from build123d import *
from build123d.topology import SkipClean

# Parameters (mm, degrees)
SKETCH2_W           = 56
SKETCH2_H           = 61
BOSS_EXTRUDE1_DEPTH = 2
SKETCH3_W           = 46
SKETCH3_H           = 53
BOSS_EXTRUDE4_DEPTH = 2
SKETCH4_W           = 61
SKETCH4_H           = 4
BOSS_EXTRUDE5_DEPTH = 1
SKETCH5_W           = 6
SKETCH5_H           = 7
SKETCH5_R           = 1.6
BOSS_EXTRUDE7_DEPTH = 4
CUT_EXTRUDE1_DEPTH  = 1
CHAMFER1_SIZE       = 7
CHAMFER2_SIZE       = 7
CHAMFER3_SIZE       = 7
SKETCH11_R          = 3.1
CUT_EXTRUDE3_DEPTH  = 2
CHAMFER5_SIZE       = 1
BOSS_EXTRUDE8_DEPTH = 4
SKETCH13_W          = 45.8
SKETCH13_H          = 52.8
CUT_EXTRUDE4_DEPTH  = 2
CHAMFER6_SIZE       = 0.5
SKETCH14_W          = 2.229283504
SKETCH14_H          = 1.6
CUT_EXTRUDE5_DEPTH  = 0.4
CHAMFER7_SIZE       = 0.4
SKETCH15_W          = 42.8
SKETCH15_H          = 20
CUT_EXTRUDE6_DEPTH  = 2
SKETCH17_W          = 105.377924995
SKETCH17_H          = 90.385080266
SKETCH17_W_2        = 45.7
SKETCH17_H_2        = 52.7
CUT_EXTRUDE7_DEPTH  = 2
FILLET1_R           = 3
FILLET2_R           = 1


with BuildPart() as part:
    # Sketch2 → Boss-Extrude1 (new, symmetric)
    with BuildSketch(Plane(origin=(0, 0, 0), x_dir=(1, 0, 0), z_dir=(0, 1, 0))):
        with Locations((-16.78535262, 5.61968945)):
            Rectangle(SKETCH2_W, SKETCH2_H)
    extrude(amount=BOSS_EXTRUDE1_DEPTH, both=True)

    # Sketch3 → Boss-Extrude4 (add)
    with BuildSketch(Plane(origin=(0, 2, 0), x_dir=(1, 0, 0), z_dir=(0, 1, 0))):
        with Locations((-15.78535262, 5.61968945)):
            Rectangle(SKETCH3_W, SKETCH3_H)
    extrude(amount=BOSS_EXTRUDE4_DEPTH)

    # Sketch4 → Boss-Extrude5 (add)
    with BuildSketch(Plane.ZY.offset(44.78535262)):
        with Locations((-5.61968945, 0)):
            Rectangle(SKETCH4_W, SKETCH4_H)
    extrude(amount=BOSS_EXTRUDE5_DEPTH)

    # Sketch5 → Boss-Extrude7 (add)
    # profile 1 of 4: a face of its own
    with BuildSketch(Plane.XZ.offset(2)):
        with Locations((0.21464738, -39.61968945)):
            Rectangle(SKETCH5_W, SKETCH5_H)
        with Locations(Location((0.21464738, -39.61968945, 0), (0, 0, 270))):
            Circle(SKETCH5_R, mode=Mode.SUBTRACT)
    # profile 2 of 4: a face of its own
    with BuildSketch(Plane.XZ.offset(2)):
        with Locations((-34.78535262, -39.61968945)):
            Rectangle(SKETCH5_W, SKETCH5_H)
        with Locations(Location((-34.78535262, -39.61968945, 0), (0, 0, 270))):
            Circle(SKETCH5_R, mode=Mode.SUBTRACT)
    # profile 3 of 4: a face of its own
    with BuildSketch(Plane.XZ.offset(2)):
        with Locations((0.21464738, 28.38031055)):
            Rectangle(SKETCH5_W, SKETCH5_H)
        with Locations(Location((0.21464738, 28.38031055, 0), (0, 0, 270))):
            Circle(SKETCH5_R, mode=Mode.SUBTRACT)
    # profile 4 of 4: a face of its own
    with BuildSketch(Plane.XZ.offset(2)):
        with Locations((-34.78535262, 28.38031055)):
            Rectangle(SKETCH5_W, SKETCH5_H)
        with Locations(Location((-34.78535262, 28.38031055, 0), (0, 0, 270))):
            Circle(SKETCH5_R, mode=Mode.SUBTRACT)
    extrude(amount=-BOSS_EXTRUDE7_DEPTH)

    # Sketch10 → Cut-Extrude1 (cut)
    with BuildSketch(Plane(origin=(0, 2, 0), x_dir=(1, 0, 0), z_dir=(0, 1, 0))):
        Polygon((6.144593809, -23.88031055), (7.179875028, -23.88031055), (10.21464738, -23.88031055), (10.21464738, 33.074495481), (10.21464738, 35.11968945), (-41.065727012, 35.11968945), (-44.18535262, 35.11968945), (-44.18535262, -21.426384345), (-44.18535262, -23.88031055), align=None)
        Polygon((5.896683614, -21.88031055), (-42.18535262, -21.88031055), (-42.18535262, 33.11968945), (8.21464738, 33.11968945), (8.21464738, -21.88031055), align=None, mode=Mode.SUBTRACT)
    extrude(amount=-CUT_EXTRUDE1_DEPTH, mode=Mode.SUBTRACT)

    # Chamfer1
    chamfer1_edges = [part.edges().sort_by_distance(p)[0] for p in [
        (3.21464738, 0, -36.11968945),
    ]]
    chamfer(chamfer1_edges, length=CHAMFER1_SIZE - 0.0001)  # a hair under: the kernel refuses the full size

    # Chamfer2
    chamfer2_edges = [part.edges().sort_by_distance(p)[0] for p in [
        (-2.78535262, 0, -36.11968945),
    ]]
    chamfer(chamfer2_edges, length=CHAMFER2_SIZE - 0.0001)  # a hair under: the kernel refuses the full size

    # Chamfer3
    chamfer3_edges = [part.edges().sort_by_distance(p)[0] for p in [
        (-37.78535262, 0, -36.11968945),
        (-31.78535262, 0, -36.11968945),
        (3.21464738, 0, 24.88031055),
        (-2.78535262, 0, 24.88031055),
        (-37.78535262, 0, 24.88031055),
        (-31.78535262, 0, 24.88031055),
    ]]
    chamfer(chamfer3_edges, length=CHAMFER3_SIZE - 0.0001)  # a hair under: the kernel refuses the full size

    # Sketch11 → Cut-Extrude3 (cut)
    with BuildSketch(Plane.XZ.offset(2)):
        with Locations(Location((-34.78535262, 28.38031055, 0), (0, 0, 270))):
            Circle(SKETCH11_R)
        with Locations(Location((0.21464738, 28.38031055, 0), (0, 0, 270))):
            Circle(SKETCH11_R)
        with Locations(Location((0.21464738, -39.61968945, 0), (0, 0, 270))):
            Circle(SKETCH11_R)
        with Locations(Location((-34.78535262, -39.61968945, 0), (0, 0, 270))):
            Circle(SKETCH11_R)
    extrude(amount=-CUT_EXTRUDE3_DEPTH, mode=Mode.SUBTRACT)

    # Chamfer5
    chamfer5_edges = [part.edges().sort_by_distance(p)[0] for p in [
        (-45.78535262, 0, -36.11968945),
        (-45.78535262, 0, 24.88031055),
        (11.21464738, 0, -36.11968945),
        (11.21464738, 0, 24.88031055),
    ]]
    chamfer(chamfer5_edges, length=CHAMFER5_SIZE)

    # Sketch12 → Boss-Extrude8 (add)
    with SkipClean():  # the faces are left unmerged after this step: merging them gives an invalid solid
        with BuildSketch(Plane.XZ.offset(2)):
            Polygon((-31.78535262, 31.88031055), (-32.78535262, 32.88031055), (-36.78535262, 32.88031055), (-37.78535262, 31.88031055), align=None)
            Polygon((3.21464738, 31.88031055), (2.21464738, 32.88031055), (-1.78535262, 32.88031055), (-2.78535262, 31.88031055), align=None)
            Polygon((-2.78535262, -43.11968945), (-1.78535262, -44.11968945), (-1.009776474, -44.11968945), (2.21464738, -44.11968945), (3.21464738, -43.11968945), align=None)
            Polygon((-31.78535262, -43.11968945), (-32.78535262, -44.11968945), (-36.78535262, -44.11968945), (-37.78535262, -43.11968945), align=None)
        extrude(amount=-BOSS_EXTRUDE8_DEPTH)

    # Sketch13 → Cut-Extrude4 (cut)
    with SkipClean():  # the faces are left unmerged after this step: merging them gives an invalid solid
        with BuildSketch(Plane(origin=(0, 4, 0), x_dir=(1, 0, 0), z_dir=(0, 1, 0))):
            Polygon((-38.78535262, -20.88031055), (-38.68535262, -20.88031055), (7.21464738, -20.88031055), (7.21464738, -20.78031055), (7.21464738, 32.01968945), (7.21464738, 32.11968945), (-38.68535262, 32.11968945), (-38.78535262, 32.11968945), align=None)
            with Locations((-15.78535262, 5.61968945)):
                Rectangle(SKETCH13_W, SKETCH13_H, mode=Mode.SUBTRACT)
        extrude(amount=-CUT_EXTRUDE4_DEPTH, mode=Mode.SUBTRACT)

    # Chamfer6
    chamfer6_edges = [part.edges().sort_by_distance(p)[0] for p in [
        (-15.78535262, 4, 20.78031055),
        (-38.68535262, 4, -5.61968945),
        (-15.78535262, 4, -32.01968945),
        (7.11464738, 4, -5.61968945),
    ]]
    chamfer(chamfer6_edges, length=CHAMFER6_SIZE)

    # Sketch14 → Cut-Extrude5 (cut)
    with SkipClean():  # the faces are left unmerged after this step: merging them gives an invalid solid
        with BuildSketch(Plane.XZ.offset(2)):
            with Locations((-40.670710868, -5.61968945)):
                Rectangle(SKETCH14_W, SKETCH14_H)
        extrude(amount=-CUT_EXTRUDE5_DEPTH, mode=Mode.SUBTRACT)

    # Chamfer7
    chamfer7_edges = [part.edges().sort_by_distance(p)[0] for p in [
        (-40.670710868, -1.6, -4.81968945),
        (-39.556069116, -1.6, -5.61968945),
        (-40.670710868, -1.6, -6.41968945),
        (-41.78535262, -1.6, -5.61968945),
    ]]
    chamfer(chamfer7_edges, length=CHAMFER7_SIZE - 0.0001)  # a hair under: the kernel refuses the full size

    # Sketch15 → Cut-Extrude6 (cut)
    with SkipClean():  # the faces are left unmerged after this step: merging them gives an invalid solid
        with BuildSketch(Plane(origin=(0, 4, 0), x_dir=(1, 0, 0), z_dir=(0, 1, 0))):
            with Locations((-15.78535262, -9.28031055)):
                Rectangle(SKETCH15_W, SKETCH15_H)
        extrude(amount=-CUT_EXTRUDE6_DEPTH, mode=Mode.SUBTRACT)

    # Sketch17 → Cut-Extrude7 (cut)
    with SkipClean():  # the faces are left unmerged after this step: merging them gives an invalid solid
        with BuildSketch(Plane(origin=(0, 4, 0), x_dir=(1, 0, 0), z_dir=(0, 1, 0))):
            with Locations((-12.998639351, 5.588523168)):
                Rectangle(SKETCH17_W, SKETCH17_H)
            with Locations((-15.78535262, 5.61968945)):
                Rectangle(SKETCH17_W_2, SKETCH17_H_2, mode=Mode.SUBTRACT)
        extrude(amount=-CUT_EXTRUDE7_DEPTH, mode=Mode.SUBTRACT)

    # Fillet1
    fillet1_edges = [part.edges().sort_by_distance(p)[0] for p in [
        (-44.18535262, 1.5, 23.88031055),
        (-44.18535262, 1.5, -35.11968945),
        (10.21464738, 1.5, -35.11968945),
        (10.21464738, 1.5, 23.88031055),
    ]]
    fillet(fillet1_edges, radius=FILLET1_R)

    # Fillet2
    fillet2_edges = [part.edges().sort_by_distance(p)[0] for p in [
        (-42.18535262, 1.5, 21.88031055),
        (-42.18535262, 1.5, -33.11968945),
        (8.21464738, 1.5, -33.11968945),
        (8.21464738, 1.5, 21.88031055),
    ]]
    fillet(fillet2_edges, radius=FILLET2_R)


solid = part.part
Model file for the job. Use its own axes, mm. A direction names the side the tool comes from. Round coordinates to 2 decimals unless told otherwise and drop trailing zeros. Loops run counter-clockwise (first coordinate to the right, second up) from the corner with the lowest first, then second, coordinate; pieces in that order, holes last. Notation, with made-up numbers: (-32, 20) - (-28, 20) arc R22 ccw to (-28, 39) - close; hole circle Ø4 at (79, 18). An arc over 180 degrees is marked (long way). Write each question's results on one line, items separated by ' | '.
(1) 3-axis set-ups, long thin cutter, end or side, ignore diameter. For faces 5 (the flat face through (0, 0, 32.88)), 6 (the cylindrical face through (-43.33, 1.49, -34.22)), 7 (the flat face through (-5.841, -0.028, 28.824)), 8 (the flat face through (-28.841, -0.028, -40.176)), 9 (the flat face through (-1, 0, -41)): which of +Z, -Z, +X, -X, +Y, -Y reach the whole face in a straight line?
Answer below:
face 5: +Z, +X, -X, +Y, -Y | face 6: +Y | face 7: +Z, +Y, -Y | face 8: -Z, +Y, -Y | face 9: -Y
(2) Saw through at A-A, the plane x = -19. List the corners of the cut face in (y, z).
Answer below:
outline: (-2, -36.12) - (2, -36.12) - (2, -35.12) - (1, -35.12) - (1, -33.12) - (2, -33.12) - (2, -31.97) - (3.55, -31.97) - (4, -31.52) - (4, -0.72) - (2, -0.72) - (2, 19.28) - (4, 19.28) - (4, 20.28) - (3.55, 20.73) - (2, 20.73) - (2, 21.88) - (1, 21.88) - (1, 23.88) - (2, 23.88) - (2, 24.88) - (-2, 24.88) - close
(3) Wall check: L1, parallel to Z at x = -7, y = 2.75; L2, parallel to Z at x = 1, y = -1.5; L3, parallel to Z at x = -36, y = 1.75. Give the ranges that are in metal, low to high.
Answer below:
L1: z = -31.97 to -0.72, 19.28 to 20.73 | L2: z = -44.12 to -42.62, -36.62 to 25.38, 31.38 to 32.88 | L3: z = -44.12 to -40.66, -38.58 to -35.12, -33.12 to 21.88, 23.88 to 27.34, 29.42 to 32.88
(4) Saw through at C-C, the plane z = -17. List the corners of the cut face in (x, y).
Answer below:
outline: (-45.79, -2) - (11.21, -2) - (11.21, 2) - (10.21, 2) - (10.21, 1) - (8.21, 1) - (8.21, 2) - (7.06, 2) - (7.06, 3.55) - (6.61, 4) - (-38.19, 4) - (-38.64, 3.55) - (-38.64, 2) - (-42.19, 2) - (-42.19, 1) - (-44.19, 1) - (-44.19, 2) - (-45.79, 2) - close
(5) Mould opens along X. For faces 1 (the flat face through (-40.729, -0.028, 28.936)), 2 (the cylindrical face through (1.146, -1.014, 25.423)), 3 (the flat face through (-40, 2, -6)), 4 (the flat face through (-5.841, -0.028, -40.064)) say: released by +X, released by -X, zero draft, split by the parting line, or undercut.
Answer below:
face 1: released by -X | face 2: undercut | face 3: zero draft | face 4: undercut
(6) Saw through at B-B, the plane z = 1. List the corners of the cut face in (x, y).
Answer below:
outline: (-45.79, -2) - (11.21, -2) - (11.21, 2) - (10.21, 2) - (10.21, 1) - (8.21, 1) - (8.21, 2) - (7.06, 2) - (7.06, 3.55) - (6.61, 4) - (5.61, 4) - (5.61, 2) - (-37.19, 2) - (-37.19, 4) - (-38.19, 4) - (-38.64, 3.55) - (-38.64, 2) - (-42.19, 2) - (-42.19, 1) - (-44.19, 1) - (-44.19, 2) - (-45.79, 2) - close
(7) Pin check, flat tips, straight feed: pin 1 (5 mm diameter, centred on x = 0.21, z = -39.62, fed in from -Y); pin 2 (5.5 mm diameter, centred on x = 0.21, z = 28.38, fed in from +Y); pin 3 (1 mm diameter, centred on y = 3, z = -27, fed in from +X). Stop position of each tip, or through.
Answer below:
pin 1: stops at y = 0 | pin 2: stops at y = 2 | pin 3: stops at x = 7.06
